Input: part model. Units: mm. Frame: model coordinates. A direction names the side the tool comes from. Round coordinates to 2 decimals unless told otherwise and drop trailing zeros. Loops run counter-clockwise (first coordinate to the right, second up) from the corner with the lowest first, then second, coordinate; pieces in that order, holes last. Notation, with made-up numbers: (-24, -19.75) -> (33, -19.75) arc R7 cw to (33, -13.75) -> close; hole circle Ø11 at (-7, 88.25). An arc over 180 degrees is marked (long way). Answer as a JSON object with one key per item and string values.
Autodesk Inventor part; units mm, degrees
ref_plane "YZ Plane" through (0, 0, 0) normal (1, 0, 0) x (0, 1, 0)
ref_plane "XZ Plane" through (0, 0, 0) normal (0, 1, 0) x (-1, 0, 0)
ref_plane "XY Plane" through (0, 0, 0) normal (0, 0, 1) x (1, 0, 0)
sketch "スケッチ1" plane through (0, 0, 0) normal (0, 0, 1) x (1, 0, 0)
  circle A0 centre (0, 0) radius 28.5
  circle A1 centre (0, 0) radius 20
  dimension "d0" = 57
  dimension "d1" = 40
extrude "押し出し1" add sketch "スケッチ1" along normal blind 10 contours A0 | A1
sketch "スケッチ2" plane through (0, 0, 0) normal (0, 0, -1) x (-1, 0, 0)
  circle A0 centre (0, 0) radius 22.5
  dimension "d4" = 45
extrude "押し出し2" cut sketch "スケッチ2" against normal blind 5
sketch "スケッチ3" plane through (0, 0, 5) normal (0, 0, -1) x (-1, 0, 0)
  circle A0 centre (0, 0) radius 19.6
  circle A1 centre (19.6, 0) radius 1.4
  circle A2 centre (0, 19.6) radius 1.4
  circle A3 centre (-19.6, 0) radius 1.4
  circle A4 centre (0, -19.6) radius 1.4
  dimension "d7" = 39.2
  dimension "d8" = 2.8
  dimension "d11" = 360
extrude "押し出し3" cut sketch "スケッチ3" against normal blind 5 contours A0 A1 | A0 A1 | A2 A0 | A0 A2 | A4 A0 | A0 A4 | A3 A0 | A0 A3
sketch "スケッチ4" plane through (0, 0, 10) normal (0, 0, 1) x (1, 0, 0)
  circle A0 centre (0, 0) radius 25
  circle A1 centre (0, -25) radius 1.7
  circle A2 centre (21.6506, -12.5) radius 1.7
  circle A3 centre (21.6506, 12.5) radius 1.7
  circle A4 centre (0, 25) radius 1.7
  circle A5 centre (-21.6506, 12.5) radius 1.7
  circle A6 centre (-21.6506, -12.5) radius 1.7
  dimension "d15" = 50
  dimension "d16" = 3.4
  dimension "d19" = 360
extrude "押し出し4" cut sketch "スケッチ4" against normal blind 10 contours A3 A0 | A0 A3 | A2 A0 | A0 A2 | A4 A0 | A0 A4 | A1 A0 | A0 A1 | A5 A0 | A0 A5 | A6 A0 | A0 A6
sketch "スケッチ5" plane through (0, 0, 10) normal (0, 0, 1) x (1, 0, 0)
  circle A0 centre (0, 0) radius 28.5
extrude "押し出し5" cut sketch "スケッチ5" against normal blind 3
sketch "スケッチ6" plane through (0, 0, 7) normal (0, 0, 1) x (1, 0, 0)
  circle A0 centre (0, 0) radius 21.5
  circle A1 centre (0, 25) radius 1.7
  circle A2 centre (0, 25) radius 3
  circle A3 centre (-21.6506, 12.5) radius 3
  circle A4 centre (-21.6506, -12.5) radius 3
  circle A5 centre (0, -25) radius 3
  circle A6 centre (21.6506, -12.5) radius 3
  circle A7 centre (21.6506, 12.5) radius 3
  dimension "d25" = 43
  dimension "d26" = 6
  dimension "d29" = 360
extrude "押し出し6" cut sketch "スケッチ6" against normal blind 1.5 contours A1 | A2 | A3 | A4 | A5 | A6 | A7
properties part number "piper-GIM3505-8" material "ABS プラスチック"
1) Section D-D, the plane y = -19.6. Output: boundary loops of the cut face in (x, z).
Output:
{"outline": "(-20.69, 0) -> (-11.05, 0) -> (-11.05, 5) -> (-1.4, 5) -> (-1.4, 7) -> (-20.69, 7) -> close; (1.4, 5) -> (11.05, 5) -> (11.05, 0) -> (20.69, 0) -> (20.69, 7) -> (1.4, 7) -> close"}
2) Section B-B, the plane z = 3. Output: boundary loops of the cut face in (x, y), plus the area to 3 significant figures.
Output:
{"outline": "circle Ø57 at (0, 0); hole circle Ø3.4 at (-21.65, -12.5); hole circle Ø3.4 at (-21.65, 12.5); hole circle Ø45 at (0, 0); hole circle Ø3.4 at (0, -25); hole circle Ø3.4 at (0, 25); hole circle Ø3.4 at (21.65, -12.5); hole circle Ø3.4 at (21.65, 12.5)", "area": "907 mm^2"}
3) Section A-A, the plane x = 0. Count the separate pieces of the cut face and the enclosed holes in it, plus the area to 3 significant figures.
Output:
{"separate pieces": "5", "enclosed holes": "0", "area": "107 mm^2"}
4) Draft query along Y for faces 1 (the face through (0, 0, 7)), 2 (the face through (26.327, 10.916, 3.451)), 3 (the face through (-20, 11, 5.5)). Return one class per face: +Y half, -Y half, draft (parallel to the pull), parting line (faces both ways), or undercut.
Output:
{"face 1": "draft", "face 2": "parting line", "face 3": "undercut"}
5) Section C-C, the plane y = 0. Output: boundary loops of the cut face in (x, z).
Output:
{"outline": "(-28.5, 0) -> (-22.5, 0) -> (-22.5, 5) -> (-21, 5) -> (-21, 7) -> (-28.5, 7) -> close; (-18.2, 5) -> (18.2, 5) -> (18.2, 7) -> (-18.2, 7) -> close; (21, 5) -> (22.5, 5) -> (22.5, 0) -> (28.5, 0) -> (28.5, 7) -> (21, 7) -> close"}
6) Contact query for flat-ended pins moving along their axis: P1, Ø4, axis at y = 3, z = 5.5, coming from the +X side; P2, Ø5.5, axis at x = 0, y = -25, coming from the +Z side; P3, Ø2, axis at y = 16, z = 3.5, coming from the -X side. Output: stop coordinate, or through.
Output:
{"P1": "stops at x = 28.48", "P2": "stops at z = 5.5", "P3": "stops at x = -24.23"}
7) Reachability of faces 4 (the face through (-0.65, 22.07, 6.26)), 5 (the face through (-10.382, -19.961, 2.465)), 6 (the face through (-20.03, 13.01, 2.79)) from +Z, -Z, +X, -X, +Y, -Y: full face, straight path, thin tool, end or side. Return the list, or none.
Output:
{"face 4": "+Z", "face 5": "-Z", "face 6": "+Z, -Z"}
8) Ray query, probe 1 along Y at (x, z) = (0, 2.6); probe 2 along X at (y, z) = (0.5, 1.5); probe 3 along Y at (x, z) = (-1, 3.75). Return the intervals inside material, ascending.
Output:
{"probe 1": "y = -28.5 to -26.7, -23.3 to -22.5, 22.5 to 23.3, 26.7 to 28.5", "probe 2": "x = -28.5 to -22.49, 22.49 to 28.5", "probe 3": "y = -28.48 to -26.37, -23.63 to -22.48, 22.48 to 23.63, 26.37 to 28.48"}
